The model under review builds one solid part; all positions refer to its coordinate system, in mm. A direction names the side the tool comes from. Round coordinates to 2 decimals unless told otherwise and drop trailing zeros. Loops run counter-clockwise (first coordinate to the right, second up) from the corner with the lowest first, then second, coordinate; pieces in that order, holes last. Notation, with made-up numbers: (-34, 67) - (-4, 67) arc R15 cw to (-4, 79) - close; hole circle Ø4 at (-30.75, 48.25). An arc over 180 degrees is marked (long way). Answer as CSV lines item,"result".
Autodesk Inventor part; units mm, degrees
ref_plane "工作平面1" through (0, 15, 105) normal (0, 1, 0) x (-1, 0, 0)
ref_plane "YZ Plane" through (0, 0, 0) normal (1, 0, 0) x (0, 1, 0)
ref_plane "XY Plane" through (0, 0, 0) normal (0, 0, 1) x (1, 0, 0)
sketch "草图1" plane through (0, 0, 0) normal (0, 0, 1) x (1, 0, 0)
  circle A0 centre (0, 0) radius 32
  dimension "d0" = 64
extrude "拉伸1" add sketch "草图1" along normal blind 25
sketch "草图2" plane through (0, 0, 25) normal (0, 0, 1) x (1, 0, 0)
  circle A0 centre (0, 0) radius 20
  dimension "d3" = 40
extrude "拉伸2" add sketch "草图2" along normal blind 80
sketch "草图3" plane through (0, 0, 0) normal (0, 0, -1) x (-1, 0, 0)
  circle A0 centre (0, 0) radius 25
  dimension "d6" = 50
extrude "拉伸3" add sketch "草图3" along normal blind 535
sketch "草图4" plane through (0, 0, -535) normal (0, 0, -1) x (-1, 0, 0)
  circle A0 centre (0, 0) radius 20
  dimension "d9" = 40
extrude "拉伸4" add sketch "草图4" along normal blind 30
chamfer "倒角1" distance 2 angle 45 1 edges at (20, 0, -565)
sketch "草图5" plane through (0, 0, -535) normal (0, 0, -1) x (-1, 0, 0)
  circle A0 centre (0, 0) radius 25
  circle A1 centre (0, 0) radius 20
  line L0 (-4, 24.6779) -> (-4, 19.5959)
  line L1 (4, 24.6779) -> (4, 19.5959)
  circle A2 centre (0, 0) radius 20
  circle A3 centre (0, 0) radius 25
  line L2 (0, 0) -> (0, 7.2531)
  line L3 (-19.3717, 15.8031) -> (-14.9706, 13.2621)
  line L4 (-23.3717, -8.8749) -> (-18.9706, -6.3339)
  line L5 (-4, -24.6779) -> (-4, -19.5959)
  line L6 (19.3717, -15.8031) -> (14.9706, -13.2621)
  line L7 (23.3717, 8.8749) -> (18.9706, 6.3339)
  line L8 (-14.9706, 13.2621) -> (-19.3717, 15.8031)
  arc A4 (-4, 24.6779) -> (-19.3717, 15.8031) centre (0, 0) ccw
  arc A5 (-4, 19.5959) -> (-14.9706, 13.2621) centre (0, 0) ccw
  dimension "d15" = 50
  dimension "d16" = 40
  dimension "d17" = 7.2531
  dimension "d18" = 4
  dimension "d19" = 8
  dimension "d22" = 360
extrude "拉伸5" cut sketch "草图5" against normal blind 505 contours L0 A1 L3 A0
pattern_circular "环形阵列1" count 6 over 360 about axis through (0, 0, -10) along (0, 0, 1) of "拉伸5"
sketch "草图6" plane through (0, 0, 105) normal (0, 0, 1) x (1, 0, 0)
  circle A0 centre (0, 0) radius 15
  circle A1 centre (0, 0) radius 20
  dimension "d29" = 30
  dimension "d30" = 40
extrude "拉伸6" cut sketch "草图6" against normal blind 28.578
sketch "草图7" plane through (0, 0, 0) normal (0, 1, 0) x (-1, 0, 0)
  line L0 (-13.95, 99.352) -> (-18.95, 99.352)
  line L1 (-18.95, 99.352) -> (-18.95, 100.752)
  line L2 (-18.95, 100.752) -> (-13.95, 100.752)
  line L3 (-13.95, 100.752) -> (-13.95, 99.352)
  line L4 (0, 0) -> (0, 169.8002)
  line L5 (15, 105) -> (-15, 105)
  line L6 (0, -711.96) -> (0, 316.7602)
  dimension "d33" = 169.8002
  dimension "d34" = 13.95
  dimension "d35" = 4.248
  dimension "d36" = 1.4
  dimension "d37" = 5
revolve "旋转1" cut sketch "草图7" angle 360 about axis through (0, 0, -10) along (0, 0, 1)
ref_plane "工作平面1" through (0, 15, 105) normal (0, 1, 0) x (-1, 0, 0)
sketch "草图8" plane through (0, 15, 105) normal (0, 1, 0) x (-1, 0, 0)
  line L0 (4, -22.237) -> (-4, -22.237)
  line L1 (-4, -22.237) -> (-4, -12.237)
  line L2 (-4, -12.237) -> (4, -12.237)
  line L3 (4, -12.237) -> (4, -22.237)
  arc A0 (-4, -22.237) -> (4, -22.237) centre (0, -22.237) ccw
  arc A1 (4, -12.237) -> (-4, -12.237) centre (0, -12.237) ccw
  line L4 (-15, -5.648) -> (15, -5.648)
  line L5 (15, 0) -> (-15, 0)
  line L6 (0, 0) -> (0, 18.2304)
  point P0 (0, -105)
  dimension "d39" = 8
  dimension "d40" = 10
  dimension "d41" = 6.589
  dimension "d42" = 18.2304
extrude "拉伸7" cut sketch "草图8" against normal blind 3
properties part number "主动轴"
1. Tool access review of faces 1 (the face through (0, 0, 105)), 2 (the face through (-19.1, -16.4, 0)), 3 (the face through (-4.336, 19.524, 50.351)), 4 (the face through (-3.02, 13.62, 100.04)): name each direction out of +Z, -Z, +X, -X, +Y, -Y from which nothing blocks a thin tool from reaching the whole face with its end or side.
Numbers:
face 1,"+Z, +X, -X, +Y, -Y"
face 2,"-Z"
face 3,"+Z"
face 4,"none"
2. Draft analysis for pull direction Z (two halves, no side actions). For faces 5 (the face through (14, 15, 25)), 6 (the face through (10, -10, 99.352)), 7 (the face through (-6.94, 31.24, 12.32)), state which applies: +Z half, -Z half, draft (parallel to the pull), parting line (faces both ways), or undercut.
Numbers:
face 5,"+Z half"
face 6,"undercut"
face 7,"draft"
3. Take a section at A-A (z = -444). State the section outline as (x, y) points.
Numbers:
outline,"(-23.37, -8.87) arc R25 ccw to (-19.37, -15.8) - (-14.97, -13.26) arc R20 ccw to (-4, -19.6) - (-4, -24.68) arc R25 ccw to (4, -24.68) - (4, -19.6) arc R20 ccw to (14.97, -13.26) - (19.37, -15.8) arc R25 ccw to (23.37, -8.87) - (18.97, -6.33) arc R20 ccw to (18.97, 6.33) - (23.37, 8.87) arc R25 ccw to (19.37, 15.8) - (14.97, 13.26) arc R20 ccw to (4, 19.6) - (4, 24.68) arc R25 ccw to (-4, 24.68) - (-4, 19.6) arc R20 ccw to (-14.97, 13.26) - (-19.37, 15.8) arc R25 ccw to (-23.37, 8.87) - (-18.97, 6.33) arc R20 ccw to (-18.97, -6.33) - close"
4. Clearance check with flat-ended pins moving along their axes: pin 1 (5 mm diameter, centred on x = -21, y = 2, fed in from -Z) (3 decimals); pin 2 (4 mm diameter, centred on x = 21, y = -9.5, fed in from -Z); pin 3 (8 mm diameter, centred on x = -22.5, y = -15, fed in from +Z). State where each tip first meets the part, or that it passes through.
Numbers:
pin 1,"stops at z = -564.405"
pin 2,"stops at z = -535"
pin 3,"stops at z = 25"
5. Wall thickness on probe 1 along X at (y, z) = (-15, -497.5); probe 2 along X at (y, z) = (-14, -224); probe 3 along Z at (x, y) = (21.5, 11.5): over which ranges is each line inside the solid? List them lowest first.
Numbers:
probe 1,"x = -20 to -17.98, -13.23 to 13.23, 17.98 to 20"
probe 2,"x = -20.71 to -16.25, -14.28 to 14.28, 16.25 to 20.71"
probe 3,"z = -535 to 25"
